from build123d import *

# Parameters (mm, degrees)
SKETCH1_W           = 80
SKETCH1_H           = 160
BOSS_EXTRUDE1_DEPTH = 56
SHELL1_T            = -3
SKETCH2_W           = 40
SKETCH2_H           = 30
CUT_EXTRUDE1_DEPTH  = 70
SKETCH4_W           = 70
SKETCH4_H           = 15
CUT_EXTRUDE3_DEPTH  = 70
SKETCH5_W           = 20
SKETCH5_H           = 10
SKETCH5_R           = 2
BOSS_EXTRUDE2_DEPTH = 3
SKETCH6_R           = 2
CUT_EXTRUDE4_DEPTH  = 3
FILLET1_R           = 3


with BuildPart() as part:
    # Sketch1 → Boss-Extrude1 (new body)
    with BuildSketch(Plane.XY):
        Rectangle(SKETCH1_W, SKETCH1_H)
    extrude(amount=BOSS_EXTRUDE1_DEPTH)

    # Shell1
    shell1_openings = [part.faces().sort_by_distance(p)[0] for p in [
        (0, 0, 0),
    ]]
    offset(amount=SHELL1_T, openings=shell1_openings, kind=Kind.INTERSECTION)

    # Sketch2 → Cut-Extrude1 (cut)
    with BuildSketch(Plane(origin=(0, 80, 0), x_dir=(1, 0, 0), z_dir=(0, 1, 0))):
        with Locations((0, -26)):
            Rectangle(SKETCH2_W, SKETCH2_H)
    extrude(amount=-CUT_EXTRUDE1_DEPTH, mode=Mode.SUBTRACT)

    # Sketch4 → Cut-Extrude3 (cut)
    with BuildSketch(Plane(origin=(0, -80, 0), x_dir=(-1, 0, 0), z_dir=(0, -1, 0))):
        with Locations((0, -7.5)):
            Rectangle(SKETCH4_W, SKETCH4_H)
    extrude(amount=-CUT_EXTRUDE3_DEPTH, mode=Mode.SUBTRACT)

    # Sketch5 → Boss-Extrude2 (add)
    # profile 1 of 2: a face of its own
    with BuildSketch(Plane(origin=(0, 0, 0), x_dir=(-1, 0, 0), z_dir=(0, 0, -1))):
        with Locations((50, 60)):
            Rectangle(SKETCH5_W, SKETCH5_H)
        with Locations((55, 60)):
            Circle(SKETCH5_R, mode=Mode.SUBTRACT)
    # profile 2 of 2: a face of its own
    with BuildSketch(Plane(origin=(0, 0, 0), x_dir=(-1, 0, 0), z_dir=(0, 0, -1))):
        with Locations((50, -70)):
            Rectangle(SKETCH5_W, SKETCH5_H)
        with Locations((55, -70)):
            Circle(SKETCH5_R, mode=Mode.SUBTRACT)
    boss_extrude2 = extrude(amount=-BOSS_EXTRUDE2_DEPTH)

    # Mirror1: Boss-Extrude2 across plane
    add(boss_extrude2.mirror(Plane(origin=(0, 0, 0), x_dir=(0, 0, 1), z_dir=(1, 0, 0))))

    # Sketch6 → Cut-Extrude4 (cut)
    with BuildSketch(Plane(origin=(0, 80, 0), x_dir=(1, 0, 0), z_dir=(0, 1, 0))):
        with Locations(Location((-27.5, -4, 0), (0, 0, 270))):
            Circle(SKETCH6_R)
        with Locations(Location((27.5, -4, 0), (0, 0, 270))):
            Circle(SKETCH6_R)
        with Locations(Location((27.5, -49, 0), (0, 0, 270))):
            Circle(SKETCH6_R)
        with Locations(Location((-27.5, -49, 0), (0, 0, 270))):
            Circle(SKETCH6_R)
    extrude(amount=-CUT_EXTRUDE4_DEPTH, mode=Mode.SUBTRACT)

    # Fillet1
    fillet1_edges = [part.edges().sort_by_distance(p)[0] for p in [
        (40, 55, 1.5),
        (60, 55, 1.5),
        (60, 65, 1.5),
        (40, -65, 1.5),
        (40, -75, 1.5),
        (60, -75, 1.5),
        (60, -65, 1.5),
        (-35, -78.5, 15),
        (35, -78.5, 15),
        (-40, 55, 1.5),
        (-40, 65, 1.5),
        (-60, 65, 1.5),
        (-60, 55, 1.5),
        (-40, -75, 1.5),
        (-40, -65, 1.5),
        (-60, -65, 1.5),
        (-60, -75, 1.5),
        (40, 65, 1.5),
    ]]
    fillet(fillet1_edges, radius=FILLET1_R)


solid = part.part
Build history of the part. All positions in model axes, mm. A direction names the side the tool comes from. Coordinates: 2 decimals unless noted, no trailing zeros. Write each loop counter-clockwise with the first axis right and the second up, starting at its lowest first coordinate (ties: lowest second). Pieces come first, ordered by that corner, then holes. Notation, with made-up numbers: (5, -25.5) -> (55, -25.5) arc R36 cw to (55, 12.5) -> close; hole circle Ø10 at (-8, 15). An arc over 180 degrees is marked (long way). Use CSV: the item, a comma, the result in double quotes. Start each with the question number.
Q1. Pull direction X, two halves, no side cores. Call faces 1 (the flat face through (-1, -80, 34)), 2 (the cylindrical face through (25.548, 78.521, 48.566)), 3 (the flat face through (-40, -1, 28)), 4 (the flat face through (-37, -1, 26)): released by +X, released by -X, zero draft, split by the parting line, or undercut.
Q2. Flat gauge pins, fed straight in: pin 1 Ø3.5 at (x, z) = (-52, 2) entering from +Y; pin 2 Ø1.5 at (x, y) = (-3.5, -52) entering from -Z; pin 3 Ø1.5 at (y, z) = (29, 22) entering from +X. Where does each tip first touch, or does it go through?
Q3. Cut at D-D, the plane x = 2.5. List the corners of the cut face in (y, z).
Q4. Drill centre lines: probe 1 along Y at (x, z) = (-55, 1); probe 2 along X at (y, z) = (78.3, 49); probe 3 along X at (y, z) = (-65.5, 7). Where is each one in solid material? Low to high.
Q5. Cut at A-A, the plane x = 55. List the corners of the cut face in (y, z).
Q6. Cut at C-C, the plane y = 60. List the corners of the cut face in (x, z).
Q7. 3-axis set-ups, long thin cutter, end or side, ignore diameter. For faces 5 (the flat face through (-1, 1, 53)), 6 (the flat face through (50, 60, 3)), 7 (the flat face through (-50, 60, 3)): which of +Z, -Z, +X, -X, +Y, -Y reach the whole face in a straight line?
Q8. Cut at B-B, the plane z = 49. List the corners of the cut face in (x, y), then the cut area to 3 significant figures.
Checked values:
1,face 1,"zero draft"
1,face 2,"undercut"
1,face 3,"released by -X"
1,face 4,"undercut"
2,pin 1,"stops at y = 65"
2,pin 2,"stops at z = 53"
2,pin 3,"stops at x = 40"
3,outline,"(-80, 15) -> (-77, 15) -> (-77, 53) -> (77, 53) -> (77, 41) -> (80, 41) -> (80, 56) -> (-80, 56) -> close; (77, 0) -> (80, 0) -> (80, 11) -> (77, 11) -> close"
4,probe 1,"y = -75 to -72, -68 to -65, 55 to 58, 62 to 65"
4,probe 2,"x = -40 to -29.5, -25.5 to 25.5, 29.5 to 40"
4,probe 3,"x = -40 to -37, 37 to 40"
5,outline,"(-75, 0) -> (-72, 0) -> (-72, 3) -> (-75, 3) -> close; (-68, 0) -> (-65, 0) -> (-65, 3) -> (-68, 3) -> close; (55, 0) -> (58, 0) -> (58, 3) -> (55, 3) -> close; (62, 0) -> (65, 0) -> (65, 3) -> (62, 3) -> close"
6,outline,"(-60, 0) -> (-57, 0) -> (-57, 3) -> (-60, 3) -> close; (-53, 0) -> (-37, 0) -> (-37, 53) -> (37, 53) -> (37, 0) -> (53, 0) -> (53, 3) -> (40, 3) -> (40, 56) -> (-40, 56) -> (-40, 3) -> (-53, 3) -> close; (57, 0) -> (60, 0) -> (60, 3) -> (57, 3) -> close"
7,face 5,"-Z"
7,face 6,"+Z, +X, +Y, -Y"
7,face 7,"+Z, -X, +Y, -Y"
8,outline,"(-40, -80) -> (40, -80) -> (40, 80) -> (29.5, 80) -> (29.5, 77) -> (37, 77) -> (37, -77) -> (-37, -77) -> (-37, 77) -> (-29.5, 77) -> (-29.5, 80) -> (-40, 80) -> close; (-25.5, 77) -> (25.5, 77) -> (25.5, 80) -> (-25.5, 80) -> close"
8,area,"1,380 mm²"
